Here's how the part is built. I have some questions about the finished solid (model axes, mm). Coordinates: 2 decimals unless noted, no trailing zeros. Order: outer loops, then holes, each group sorted by start corner. A loop starts at its lowest first (then second) coordinate and runs counter-clockwise, first axis right, second up. Notation, with made-up numbers: M -20.5,61.5 L 38.5,61.5 A30 cw 38.5,86.5 Z; hole C 26.25,67.5 d6. An arc over 180 degrees is marked long. One line per question, with ' | ' between items. Start each with the question number.
```python
from build123d import *

# Parameters (mm, degrees)
F0_W     = 609.6
F0_H     = 50.8
F1_DEPTH = 6.35
F2_W     = 609.6
F2_H     = 40.64
F3_DEPTH = 3.175
F4_W     = 2.032
F4_H     = 3.175
F5_DEPTH = 50.8


with BuildPart() as f1:
    # F0 (on Top) → F1 (new body)
    with BuildSketch(Plane.XY):
        Rectangle(F0_W, F0_H)
    extrude(amount=F1_DEPTH)

    # F2 (on face) → F3 (cut)
    with BuildSketch(Plane.XY.offset(6.35)):
        Rectangle(F2_W, F2_H)
    extrude(amount=-F3_DEPTH, mode=Mode.SUBTRACT)

    # F4 (on face) → F5 (cut, through all)
    with BuildSketch(Plane.XZ.offset(25.4)):
        with Locations((0, 4.7625)):
            Rectangle(F4_W, F4_H)
    extrude(amount=-F5_DEPTH, mode=Mode.SUBTRACT)


solid = f1.part
```
1. Imagine slicing it at B-B (x = 31). List the corners of the cut face in (y, z) for me (3 decimals).
2. I need wall thicknesses on line 1 (Y direction, x = 119.5, z = 6.25); line 2 (Z direction, x = -270.5, y = 17.5) (3 decimals). Which ranges of each line are inside material? Lowest first, please.
3. Imagine slicing it at A-A (z = 4.75). List the corners of the cut face in (x, y) for me, then the cut area to 3 significant figures.
4. Imagine slicing it at C-C (y = 8.5). List the corners of the cut face in (x, z) for me (3 decimals), then the cut area to 3 significant figures.
5. Will this pin go through, and if not, where does the flat tip stop? pin 1 (6 mm diameter, centred on x = -0.5, y = -9, fed in from +Z) (3 decimals).
6. We'd pull the mould along Y, two halves only. Please class faces 1 (the face through (-4, 0, 0)), 2 (the face through (-4, 0, 3.175)): released by +Y, released by -Y, zero draft, split by the parting line, or undercut.
Entries:
1) outline: M -25.4,0 L 25.4,0 L 25.4,6.35 L 20.32,6.35 L 20.32,3.175 L -20.32,3.175 L -20.32,6.35 L -25.4,6.35 Z
2) line 1: -25.4 to -20.32, 20.32 to 25.4 | line 2: 0 to 3.175
3) outline: M -304.8,-25.4 L -1.02,-25.4 L -1.02,-20.32 L -304.8,-20.32 Z; M -304.8,20.32 L -1.02,20.32 L -1.02,25.4 L -304.8,25.4 Z; M 1.02,-25.4 L 304.8,-25.4 L 304.8,-20.32 L 1.02,-20.32 Z; M 1.02,20.32 L 304.8,20.32 L 304.8,25.4 L 1.02,25.4 Z | area: 6,170 mm²
4) outline: M -304.8,0 L 304.8,0 L 304.8,3.175 L -304.8,3.175 Z | area: 1,940 mm²
5) pin 1: z = 3.175
6) face 1: zero draft | face 2: undercut
